Part print with two shaded views. Sizes in mm from the minimum x, y, z corner. Coordinates: 2 decimals unless noted, no trailing zeros. Loops run counter-clockwise (first coordinate to the right, second up) from the corner with the lowest first, then second, coordinate; pieces in that order, holes last.
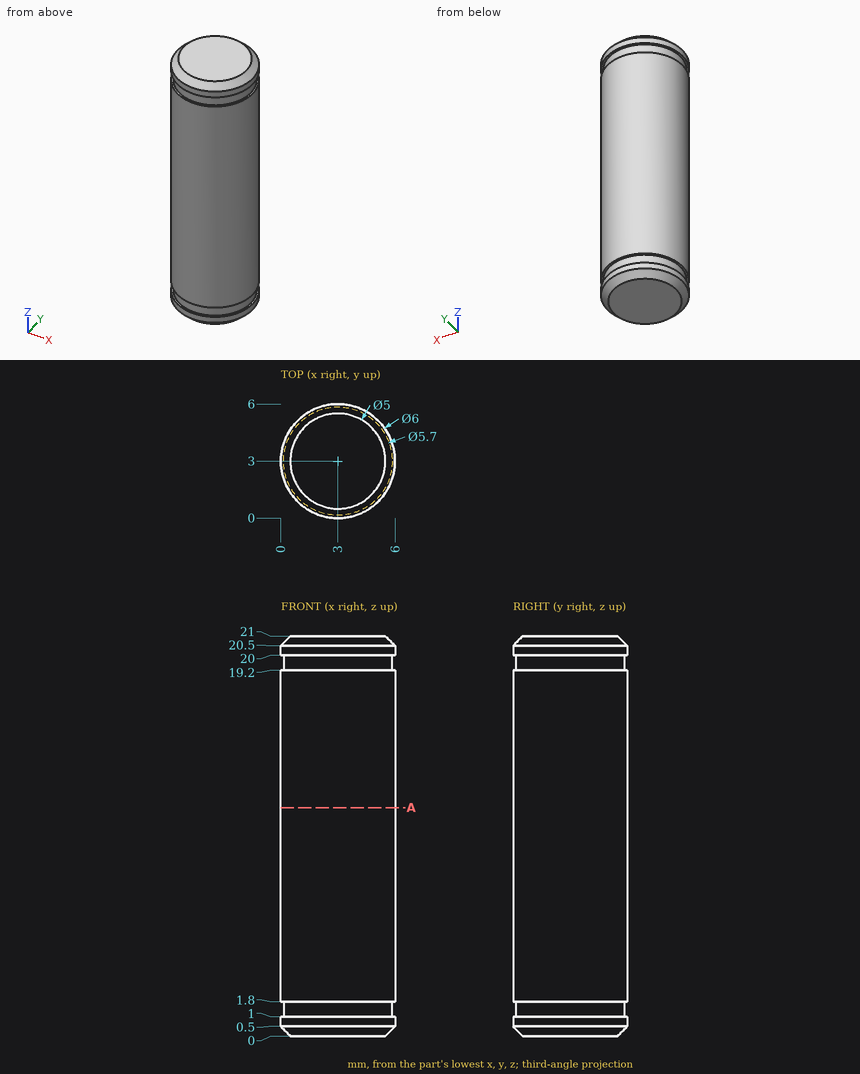
Q1. Slice it at A-A (z = 12). List the corners of the cut face in (x, y), and give its area (3 significant figures).
Answers:
outline: circle Ø6 at (3, 3)
area: 28.3 mm2
Q2. Drill centre lines: line 1 (Z direction, x = 1.2, y = 5.3); line 2 (X direction, y = 3.95, z = 16.25); line 3 (X direction, y = 3.45, z = 15). Where is each one in solid material? Low to high.
Answers:
line 1: z = 0.42 to 1, 1.8 to 19.2, 20 to 20.58
line 2: x = 0.15 to 5.85
line 3: x = 0.03 to 5.97
Q3. Flat gauge pin, fed straight in: P1, Ø3, axis at x = 1, z = 7, coming from the +Y side. Where does the tip first touch, or does it go through?
Answers:
P1: stops at y = 5.96
